from build123d import *

# Parameters (mm, degrees)
SKETCH_1_W                = 65
SKETCH_1_H                = 60
EXTRUDE_1_DEPTH           = 2
SKETCH_2_R                = 1.5
CUT_EXTRUDE_1_DEPTH       = 2
SKETCH_5_R                = 7
CUT_EXTRUDE_4_DEPTH       = 3
SKETCH_6_R                = 1.5
CUT_EXTRUDE_5_DEPTH       = 3
CUT_EXTRUDE_6_DEPTH       = 3
SKETCH_8_R                = 1.5
CUT_EXTRUDE_7_DEPTH       = 3
MIRROR_8_COPY_1_SKETCH_R  = 1.5
MIRROR_8_COPY_1_DEPTH     = 3
MIRROR_10_COPY_1_SKETCH_R = 1.5
MIRROR_10_COPY_1_DEPTH    = 2
MIRROR_10_COPY_2_SKETCH_R = 1.5
MIRROR_10_COPY_2_DEPTH    = 3
SKETCH_9_W                = 33.344360542
SKETCH_9_H                = 36.22087855
CUT_EXTRUDE_8_DEPTH       = 3
FILLET_1_R                = 2.5


with BuildPart() as part:
    # 草图1 → 凸台-拉伸1 (new body)
    with BuildSketch(Plane(origin=(0, 0, 0), x_dir=(1, 0, 0), z_dir=(0, 1, 0))):
        Rectangle(SKETCH_1_W, SKETCH_1_H)
    extrude(amount=EXTRUDE_1_DEPTH)

    # 草图2 → 切除-拉伸1 (cut)
    with BuildSketch(Plane(origin=(0, 2, 0), x_dir=(1, 0, 0), z_dir=(0, 1, 0))):
        with Locations((-28.367832783, 25)):
            Circle(SKETCH_2_R)
    cut_extrude_1 = extrude(amount=-CUT_EXTRUDE_1_DEPTH, mode=Mode.SUBTRACT)

    # 草图5 → 切除-拉伸4 (cut, through all)
    with BuildSketch(Plane(origin=(0, 2, 0), x_dir=(1, 0, 0), z_dir=(0, 1, 0))):
        Circle(SKETCH_5_R)
    extrude(amount=-CUT_EXTRUDE_4_DEPTH, mode=Mode.SUBTRACT)

    # 草图6 → 切除-拉伸5 (cut, through all)
    with BuildSketch(Plane(origin=(0, 2, 0), x_dir=(1, 0, 0), z_dir=(0, 1, 0))):
        with Locations((-28.367832783, -9)):
            Circle(SKETCH_6_R)
    cut_extrude_5 = extrude(amount=-CUT_EXTRUDE_5_DEPTH, mode=Mode.SUBTRACT)

    # 镜向7: 切除-拉伸5 across plane
    add(cut_extrude_5.mirror(Plane.XY), mode=Mode.SUBTRACT)

    # 草图7 → 切除-拉伸6 (cut, through all)
    with BuildSketch(Plane(origin=(0, 2, 0), x_dir=(1, 0, 0), z_dir=(0, 1, 0))):
        with BuildLine():
            Line((-11.509285997, 1.5), (-21.509285997, 1.5))
            ThreePointArc((-21.509285997, 1.5), (-23.009285997, 0), (-21.509285997, -1.5))
            Line((-21.509285997, -1.5), (-11.509285997, -1.5))
            ThreePointArc((-11.509285997, -1.5), (-10.009285997, 0), (-11.509285997, 1.5))
        make_face()
    cut_extrude_6 = extrude(amount=-CUT_EXTRUDE_6_DEPTH, mode=Mode.SUBTRACT)

    # 草图8 → 切除-拉伸7 (cut, through all)
    with BuildSketch(Plane(origin=(0, 2, 0), x_dir=(1, 0, 0), z_dir=(0, 1, 0))):
        with Locations((23.5, 17.75)):
            Circle(SKETCH_8_R)
    cut_extrude_7 = extrude(amount=-CUT_EXTRUDE_7_DEPTH, mode=Mode.SUBTRACT)

    # 镜向8: 切除-拉伸6, 切除-拉伸5 across plane
    add(cut_extrude_6.mirror(Plane(origin=(0, 0, 0), x_dir=(0, 0, 1), z_dir=(1, 0, 0))), mode=Mode.SUBTRACT)
    add(cut_extrude_5.mirror(Plane(origin=(0, 0, 0), x_dir=(0, 0, 1), z_dir=(1, 0, 0))), mode=Mode.SUBTRACT)

    # 镜向8 copy 1 sketch → 镜向8 copy 1 (cut, through all)
    with BuildSketch(Plane(origin=(0, 2, 0), x_dir=(-1, 0, 0), z_dir=(0, 1, 0))):
        with Locations((-28.367832783, -9)):
            Circle(MIRROR_8_COPY_1_SKETCH_R)
    extrude(amount=-MIRROR_8_COPY_1_DEPTH, mode=Mode.SUBTRACT)

    # 镜向9: 切除-拉伸1, 切除-拉伸7 across plane
    add(cut_extrude_1.mirror(Plane.XY), mode=Mode.SUBTRACT)
    add(cut_extrude_7.mirror(Plane.XY), mode=Mode.SUBTRACT)

    # 镜向10: 切除-拉伸1, 切除-拉伸7 across plane
    add(cut_extrude_1.mirror(Plane(origin=(0, 0, 0), x_dir=(0, 0, 1), z_dir=(1, 0, 0))), mode=Mode.SUBTRACT)
    add(cut_extrude_7.mirror(Plane(origin=(0, 0, 0), x_dir=(0, 0, 1), z_dir=(1, 0, 0))), mode=Mode.SUBTRACT)

    # 镜向10 copy 1 sketch → 镜向10 copy 1 (cut)
    with BuildSketch(Plane(origin=(0, 2, 0), x_dir=(-1, 0, 0), z_dir=(0, 1, 0))):
        with Locations((-28.367832783, 25)):
            Circle(MIRROR_10_COPY_1_SKETCH_R)
    extrude(amount=-MIRROR_10_COPY_1_DEPTH, mode=Mode.SUBTRACT)

    # 镜向10 copy 2 sketch → 镜向10 copy 2 (cut, through all)
    with BuildSketch(Plane(origin=(0, 2, 0), x_dir=(-1, 0, 0), z_dir=(0, 1, 0))):
        with Locations((23.5, 17.75)):
            Circle(MIRROR_10_COPY_2_SKETCH_R)
    extrude(amount=-MIRROR_10_COPY_2_DEPTH, mode=Mode.SUBTRACT)

    # 草图9 → 切除-拉伸8 (cut, through all)
    with BuildSketch(Plane(origin=(0, 2, 0), x_dir=(1, 0, 0), z_dir=(0, 1, 0))):
        with Locations((0, 30)):
            Rectangle(SKETCH_9_W, SKETCH_9_H)
    cut_extrude_8 = extrude(amount=-CUT_EXTRUDE_8_DEPTH, mode=Mode.SUBTRACT)

    # 镜向11: 切除-拉伸8 across plane
    add(cut_extrude_8.mirror(Plane.XY), mode=Mode.SUBTRACT)

    # 圆角1
    fillet_1_edges = [part.edges().sort_by_distance(p)[0] for p in [
        (16.672180271, 1, -30),
        (-16.672180271, 1, -30),
        (-16.672180271, 1, -11.889560725),
        (16.672180271, 1, -11.889560725),
        (16.672180271, 1, 30),
        (-16.672180271, 1, 30),
        (16.672180271, 1, 11.889560725),
        (-16.672180271, 1, 11.889560725),
        (-32.5, 1, -30),
        (32.5, 1, -30),
        (32.5, 1, 30),
        (-32.5, 1, 30),
    ]]
    fillet(fillet_1_edges, radius=FILLET_1_R)


solid = part.part
Verification items for the finished model (mm, model axes). A direction names the side the tool comes from. Round coordinates to 2 decimals unless told otherwise and drop trailing zeros. Order: outer loops, then holes, each group sorted by start corner. A loop starts at its lowest first (then second) coordinate and runs counter-clockwise, first axis right, second up.
1. Section check D-D on z = 9. Record the cut outline in (x, y).
Final values:
outline: (-32.5, 0) - (-29.87, 0) - (-29.87, 2) - (-32.5, 2) - close; (-26.87, 0) - (26.87, 0) - (26.87, 2) - (-26.87, 2) - close; (29.87, 0) - (32.5, 0) - (32.5, 2) - (29.87, 2) - close
2. Thickness scan on L1, parallel to Z at x = 23.5, y = 0.6; L2, parallel to X at y = 1.5, z = -25; L3, parallel to X at y = 1.55, z = 9. Record the ranges inside material, lowest first.
Final values:
L1: z = -30 to -19.25, -16.25 to 16.25, 19.25 to 30
L2: x = -32.5 to -29.87, -26.87 to -16.67, 16.67 to 26.87, 29.87 to 32.5
L3: x = -32.5 to -29.87, -26.87 to 26.87, 29.87 to 32.5
3. Go/stop test with flat-tipped pins: P1, Ø1, axis at x = 5.5, y = 0.5, coming from the -Z side; P2, Ø12, axis at x = 7, z = -24, coming from the +Y side; P3, Ø1, axis at x = -16.5, y = 1.5, coming from the -Z side; P4, Ø1, axis at x = 5, y = 1.5, coming from the +Z side. Record where each tip stops, or that it passes through.
Final values:
P1: stops at z = -11.89
P2: passes through
P3: stops at z = -28.74
P4: stops at z = 11.89
4. Section check A-A on z = 0. Record the cut outline in (x, y), then the cut area to 3 significant figures.
Final values:
outline: (-32.5, 0) - (-23.01, 0) - (-23.01, 2) - (-32.5, 2) - close; (-10.01, 0) - (-7, 0) - (-7, 2) - (-10.01, 2) - close; (7, 0) - (10.01, 0) - (10.01, 2) - (7, 2) - close; (23.01, 0) - (32.5, 0) - (32.5, 2) - (23.01, 2) - close
area: 50.0 mm2
5. Section check C-C on z = -20. Record the cut outline in (x, y), then the cut area to 3 significant figures.
Final values:
outline: (-32.5, 0) - (-16.67, 0) - (-16.67, 2) - (-32.5, 2) - close; (16.67, 0) - (32.5, 0) - (32.5, 2) - (16.67, 2) - close
area: 63.3 mm2
6. Access from +Z, -Z, +X, -X, +Y, -Y to the whole of each face (thin tool, end or side, straight path). Record for faces 1 (the cylindrical face through (15.92, 0.99, -12.6)), 2 (the flat face through (-16, 1, -1.5)), 3 (the flat face through (-16.672, 1, 21)), 4 (the flat face through (-25, 1, -30)).
Final values:
face 1: -Z, +Y, -Y
face 2: +Y, -Y
face 3: +Z, +Y, -Y
face 4: -Z, +X, -X, +Y, -Y
7. Section check B-B on x = 20. Record the cut outline in (y, z).
Final values:
outline: (0, -30) - (2, -30) - (2, -1.5) - (0, -1.5) - close; (0, 1.5) - (2, 1.5) - (2, 30) - (0, 30) - close
8. Release check for a two-part mould opening along X. For faces 5 (the cylindrical face through (-32, 1, 29)), 6 (the cylindrical face through (29.56, 1.01, -9.91)), 7 (the flat face through (25, 1, 30)) record: +X half, -X half, draft (parallel to the pull), parting line (faces both ways), or undercut.
Final values:
face 5: -X half
face 6: undercut
face 7: draft
